Geometry check sheet. Reference: the model listing, model coordinates, mm. Round coordinates to 2 decimals unless told otherwise and drop trailing zeros. Write each loop counter-clockwise with the first axis right and the second up, starting at its lowest first coordinate (ties: lowest second). Pieces come first, ordered by that corner, then holes. Notation, with made-up numbers: M 20.25,-12.75 L 65.25,-12.75 A25 cw 65.25,4.25 Z; hole C 36,52.25 d6. An arc over 180 degrees is marked long. Answer in a Markdown table with one row per item. Add a question column.
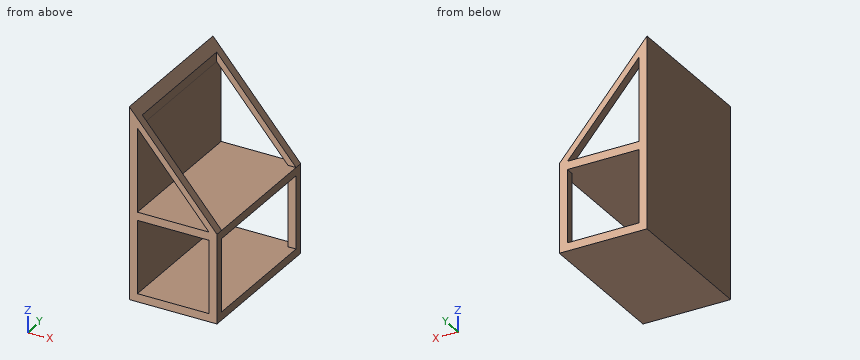
from build123d import *

# Parameters (mm, degrees)
F1_DEPTH = 180
F2_W     = 88.2857142857
F2_H     = 89.7844721901
F3_DEPTH = 294
F4_W     = 160
F4_H     = 89.7844721901
F4_H_2   = 169.9516549903
F5_DEPTH = 98


with BuildPart() as f1:
    # F0 (on Front) → F1 (new body)
    with BuildSketch(Plane.XZ):
        Polygon((-74.0419839551, 155.4725316765), (-74.0419839551, 5.1880594864), (-74.0419839551, -80.6452738469), (34.2437303306, -80.6452738469), (34.2437303306, -59.6452738469), (34.2437303306, 29.1391983432), align=None)
    extrude(amount=F1_DEPTH)

    # F2 (on face) → F3 (cut)
    with BuildSketch(Plane.XZ.offset(180)):
        Polygon((-64.0419839551, 132.1391983432), (-64.0419839551, 29.1391983432), (24.2437303306, 29.1391983432), align=None)
        with Locations((-19.8991268123, -25.7530377519)):
            Rectangle(F2_W, F2_H)
    extrude(amount=-F3_DEPTH, mode=Mode.SUBTRACT)

    # F4 (on face) → F5 (cut)
    with BuildSketch(Plane.YZ.offset(34.2437303306)):
        with Locations((-90, -25.7530377519)):
            Rectangle(F4_W, F4_H)
        with Locations((-90, 114.1150258383)):
            Rectangle(F4_W, F4_H_2)
    extrude(amount=-F5_DEPTH, mode=Mode.SUBTRACT)


solid = f1.part
Item 1: Section check A-A, the plane z = -14. Record the boundary of the cut face in (x, y).
Item 2: Gauge pin test, flat ends, axial feed: pin 1 Ø8 at (x, y) = (-10.5, -48.5) entering from +Z; pin 2 Ø6 at (y, z) = (-72, 139) entering from +X. Record the tip position at first contact, or that the pin passes through.
Item 3: Section check B-B, the plane x = -50.5. Record the boundary of the cut face in (y, z).
Item 4: Scan lines: probe 1 along Z at (x, y) = (-29, -68); probe 2 along X at (y, z) = (-127.5, 9.5); probe 3 along X at (y, z) = (-149, 134). Record each from-to range of solid material in increasing order. Write a range as from..to.
Item 5: Section check C-C, the plane y = -129. Record the boundary of the cut face in (x, z).
Result sheet:
| question | item | result |
|---|---|---|
| 1 | outline | M -74.04,-180 L -64.04,-180 L -64.04,0 L -74.04,0 Z; M 24.24,-180 L 34.24,-180 L 34.24,-170 L 24.24,-170 Z; M 24.24,-10 L 34.24,-10 L 34.24,0 L 24.24,0 Z |
| 2 | pin 1 | stops at z = 29.14 |
| 2 | pin 2 | stops at x = -63.76 |
| 3 | outline | M -180,-80.65 L 0,-80.65 L 0,-70.65 L -180,-70.65 Z; M -180,19.14 L 0,19.14 L 0,29.14 L -180,29.14 Z; M -180,116.34 L -170,116.34 L -170,128.01 L -180,128.01 Z; M -10,116.34 L 0,116.34 L 0,128.01 L -10,128.01 Z |
| 4 | probe 1 | z = -80.65..-70.65, 19.14..29.14 |
| 4 | probe 2 | x = -74.04..-64.04 |
| 4 | probe 3 | x = -74.04..-63.76 |
| 5 | outline | M -74.04,-80.65 L 34.24,-80.65 L 34.24,-70.65 L -64.04,-70.65 L -64.04,19.14 L 34.24,19.14 L 34.24,29.14 L -64.04,29.14 L -64.04,132.14 L -63.76,131.81 L -63.76,143.47 L -74.04,155.47 Z |
